Part print with two shaded views. Sizes in mm from the minimum x, y, z corner. A direction names the side the tool comes from. Round coordinates to 2 decimals unless told otherwise and drop trailing zeros. Write each loop counter-clockwise with the first axis right and the second up, starting at its lowest first coordinate (ties: lowest second). Pieces come first, ordered by that corner, then holes. Notation, with made-up numbers: (64.5, 7.5) -> (74.5, 7.5) arc R17 cw to (74.5, 32.5) -> close; hole circle Ø9 at (68.25, 30.5). An arc over 180 degrees is marked (long way). Put each result on its own line as item: value. Start each with the question number.
1. Saw through at A-A on x = 2. List the corners of the cut face in (y, z).
2. Saw through at B-B on z = 5.25. List the corners of the cut face in (x, y).
3. Saw through at D-D on x = 0.8. List the corners of the cut face in (y, z).
4. Drill centre lines: line 1 (Z direction, x = 0.9, y = 0.75); line 2 (Z direction, x = 1.5, y = 1.85); line 3 (X direction, y = 2.55, z = 5). Where is each one in solid material? Low to high. Write a range as from..to.
5. Flat gauge pins, fed straight in: P1, Ø1, axis at y = 1, z = 2, coming from the -X side; P2, Ø1, axis at x = 1, z = 6, coming from the +Y side; P3, Ø1.4, axis at x = 2, y = 2, coming from the -Z side. Where does each tip first touch, or does it go through?
6. Pull direction X, two halves, no side cores. Call the marked faces 1, 2 and 3: pulls with the +X half, pulls with the -X half, needs draft (parallel to the pull), parting line crosses it, or undercut.
7. 3-axis set-ups, long thin cutter, end or side, ignore diameter. For the marked faces 4, 5 and 6: which of +Z, -Z, +X, -X, +Y, -Y reach the whole face in a straight line?
8. Saw through at C-C on y = 1.25. List the corners of the cut face in (x, z).
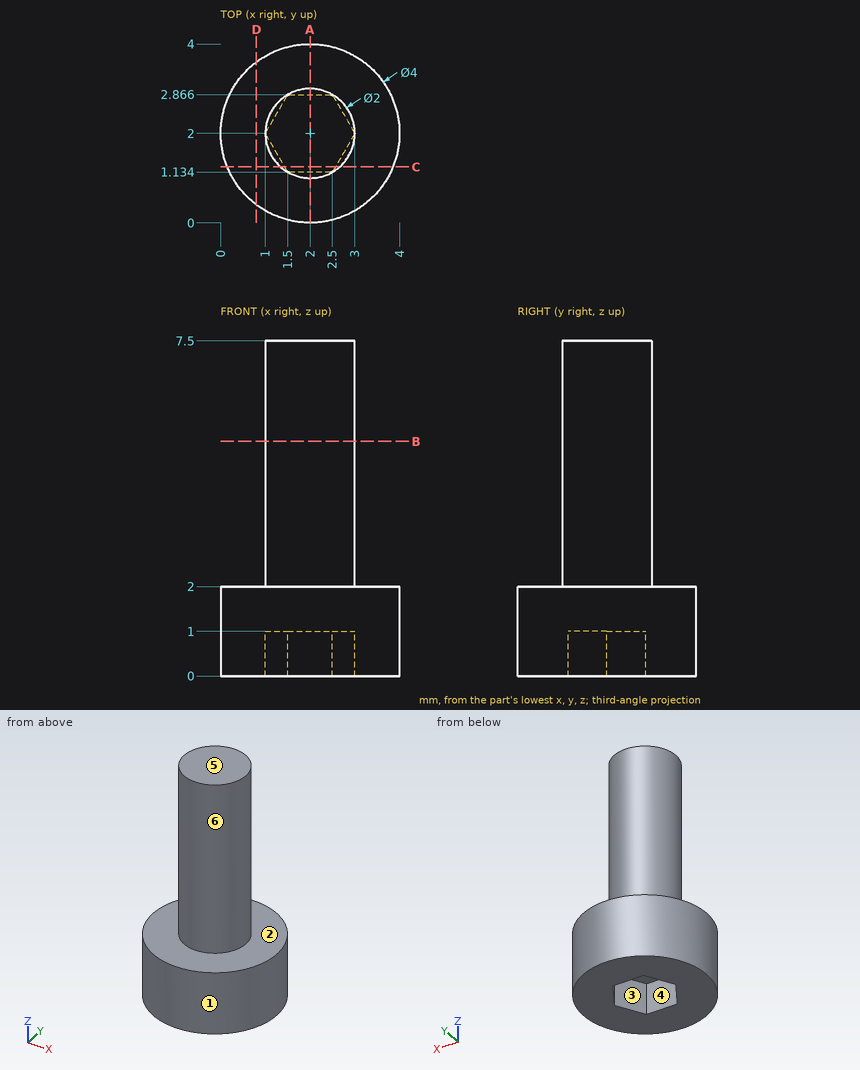
Return value:
1. outline: (0, 0) -> (1.13, 0) -> (1.13, 1) -> (2.87, 1) -> (2.87, 0) -> (4, 0) -> (4, 2) -> (3, 2) -> (3, 7.5) -> (1, 7.5) -> (1, 2) -> (0, 2) -> close
2. outline: circle Ø2 at (2, 2)
3. outline: (0.4, 0) -> (3.6, 0) -> (3.6, 2) -> (0.4, 2) -> close
4. line 1: z = 0..2
4. line 2: z = 1..7.5
4. line 3: x = 1.16..2.84
5. P1: stops at x = 0.06
5. P2: stops at y = 2.87
5. P3: stops at z = 1
6. face 1: parting line crosses it
6. face 2: needs draft
6. face 3: undercut
7. face 4: -Z
7. face 5: +Z, +X, -X, +Y, -Y
7. face 6: +Z
8. outline: (0.15, 0) -> (1.43, 0) -> (1.43, 1) -> (2.57, 1) -> (2.57, 0) -> (3.85, 0) -> (3.85, 2) -> (2.66, 2) -> (2.66, 7.5) -> (1.34, 7.5) -> (1.34, 2) -> (0.15, 2) -> close
